Could you check a few things on this model? Use its own coordinates, in mm. Face numbers are marked on the shaded views. A direction names the side the tool comes from. Round coordinates to 2 decimals unless told otherwise and drop trailing zeros. Loops run counter-clockwise (first coordinate to the right, second up) from the corner with the lowest first, then second, coordinate; pieces in that order, holes last. Notation, with made-up numbers: M 46,0 L 58,0 A16 ccw 58,7 Z; hole C -7,-23 d9. An arc over 180 degrees is marked long. One line per item, written item: value. Start each with the question number.
Q1. I'm going to push flat-ended pins straight in: pin 1 Ø16 at (x, z) = (28, 7) entering from +Y; pin 2 Ø10 at (x, z) = (24.5, -21) entering from -Y; pin 3 Ø5.5 at (y, z) = (-6, -3.5) entering from -X; pin 4 Ø8 at (x, y) = (27.5, -5.5) entering from +Z. Where does each tip first touch, or does it pass through?
Q2. Imagine slicing it at B-B (z = -7.5). Please give me the cut outline in (x, y).
Q3. Which directions (+Z, -Z, +X, -X, +Y, -Y) give clear straight access to the entire face, cutting with the end or side of a thin tool? Please do the marked faces 1, 2 and 3.
Q4. Imagine slicing it at D-D (z = 7). Please give me the cut outline in (x, y), then the cut area to 3 significant figures.
Q5. Imagine slicing it at A-A (x = 28). Please give me the cut outline in (y, z), then the cut area to 3 significant figures.
Q6. Imagine slicing it at C-C (y = -3.75). Please give me the cut outline in (x, z).
Q7. Please list where these lines run through material, in increasing order: line 1 along X through (y, z) = (-6.25, -12.5); line 2 along Y through (x, z) = (33.5, -25); line 3 along Z through (x, y) = (31, 2.75).
Q8. Thinking about a two-plate mould opening in X: for the marked faces 4, 5 and 6, which applies, released by +X, released by -X, zero draft, split by the parting line, or undercut?
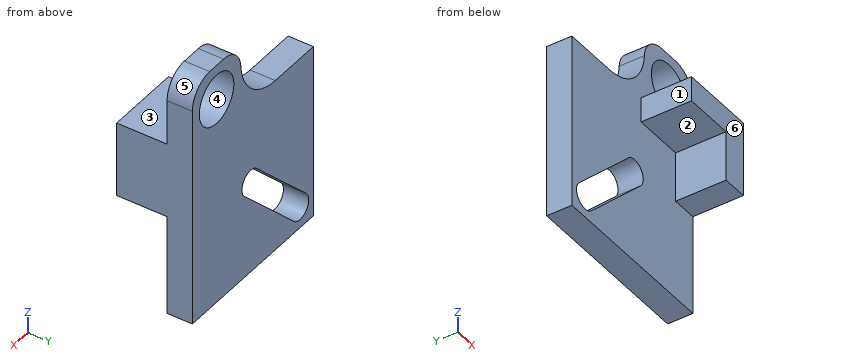
from build123d import *

# Parameters (mm, degrees)
SKETCH1_R           = 5
BOSS_EXTRUDE1_DEPTH = 5
BOSS_EXTRUDE2_DEPTH = 10
FILLET1_R           = 10
FILLET4_R           = 5


with BuildPart() as part:
    # Sketch1 → Boss-Extrude1 (new body)
    with BuildSketch(Plane(origin=(0, 0, 0), x_dir=(1, 0, 0), z_dir=(0, 1, 0))):
        Polygon((0, 0), (0, 35), (35, 35), (35, 0), (35, -14), (21, -14), (21, 0), align=None)
        with Locations(Location((28, -7, 0), (0, 0, 270))):
            Circle(SKETCH1_R, mode=Mode.SUBTRACT)
        with BuildLine():
            Line((5.77728435, 32.399644503), (19.919419974, 18.257508879))
            ThreePointArc((19.919419974, 18.257508879), (19.829534471, 14.632089471), (16.21302376, 14.901525103))
            Line((16.21302376, 14.901525103), (2.070888136, 29.043660727))
            ThreePointArc((2.070888136, 29.043660727), (2.160773638, 32.669080135), (5.77728435, 32.399644503))
        make_face(mode=Mode.SUBTRACT)
    extrude(amount=BOSS_EXTRUDE1_DEPTH)

    # Sketch2 → Boss-Extrude2 (add)
    with BuildSketch(Plane.XZ):
        Polygon((30, -5), (20, -5), (20, 0), (35, 0), (35, -15), (30, -15), align=None)
    extrude(amount=BOSS_EXTRUDE2_DEPTH)

    # Fillet1
    # the kernel refuses this fillet: 10 mm, written as the material it adds along each edge
    with BuildSketch(Plane(origin=(21, 0, 0), x_dir=(-1, 0, 0), z_dir=(0, 1, 0))) as fillet1_piece_1:
        with BuildLine():
            CenterArc((FILLET1_R, FILLET1_R), FILLET1_R, 180, 90)
            Line((0, FILLET1_R), (0, 0))
            Line((0, 0), (FILLET1_R, 0))
        make_face()
    extrude(amount=5)

    # Fillet4
    fillet4_edges = [part.edges().sort_by_distance(p)[0] for p in [
        (35, 2.5, 14),
        (21, 2.5, 14),
    ]]
    fillet(fillet4_edges, radius=FILLET4_R)


solid = part.part
Report:
1. pin 1: stops at y = 5
1. pin 2: stops at y = 0
1. pin 3: stops at x = 20
1. pin 4: stops at z = 0
2. outline: M 0,0 L 30,0 L 30,-10 L 35,-10 L 35,5 L 0,5 Z
3. face 1: +Z, -Z, -X, -Y
3. face 2: -Z, -X, -Y
3. face 3: +Z, +X, -X, -Y
4. outline: M 20.54,0 L 23,0 L 23,5 L 20.54,5 Z; M 33,0 L 35,0 L 35,5 L 33,5 Z
4. area: 22.3 mm²
5. outline: M -10,-5 L 0,-5 L 0,-35 L 5,-35 L 5,2 L 0,2 L 0,0 L -10,0 Z; M 0,12 L 5,12 L 5,14 L 0,14 Z
5. area: 245 mm²
6. outline: M 20,-5 L 30,-5 L 30,-15 L 35,-15 L 35,0 L 20,0 Z
7. line 1: x = 30 to 35
7. line 2: y = 0 to 5
7. line 3: z = -35 to 3, 11 to 13.9
8. face 4: undercut
8. face 5: released by +X
8. face 6: zero draft
